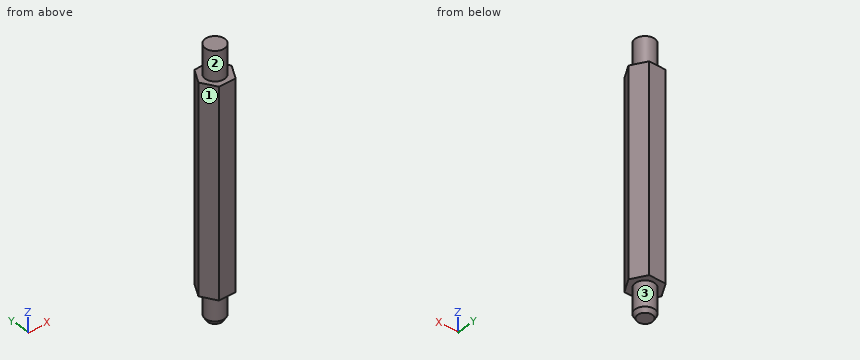
from build123d import *

# Parameters (mm, degrees)
EXTRUDE_1_DEPTH      = 42
EXTRUDE_2_DEPTH      = 6
EXTRUDE_2_DEPTH_BACK = 48
SKETCH_2_R           = 2
CHAMFER_1_SIZE       = 0.5
CHAMFER_1_SIZE2      = 0.866025404


with BuildPart() as part:
    # 草图1 → 拉伸1 (new body)
    with BuildSketch(Plane.XY):
        Polygon((1.732050808, -3), (3.464101615, 0), (1.732050808, 3), (-1.732050808, 3), (-3.464101615, 0), (-1.732050808, -3), align=None)
    extrude(amount=EXTRUDE_1_DEPTH)

    # 草图2 → 拉伸2 (add, two sides: drawn at the far end of the back side and taken through both)
    with BuildSketch(Plane.XY.offset(42).offset(-EXTRUDE_2_DEPTH_BACK)):
        with Locations(Location((0, 0, 0), (0, 0, 180))):
            Circle(SKETCH_2_R)
    extrude(amount=EXTRUDE_2_DEPTH + EXTRUDE_2_DEPTH_BACK)

    # 倒角1
    chamfer_1_edges = [part.edges().sort_by_distance(p)[0] for p in [
        (2, 0, -6),
    ]]
    chamfer_1_side = [part.faces().sort_by_distance(p)[0] for p in [
        (0, 0, -6),
    ]]
    chamfer(chamfer_1_edges, length=CHAMFER_1_SIZE, length2=CHAMFER_1_SIZE2, reference=chamfer_1_side[0])


solid = part.part
Design review of the part built by this model. Coordinates are the model's own, in mm. Face numbers are marked on the shaded views. A direction names the side the tool comes from. Round coordinates to 2 decimals unless told otherwise and drop trailing zeros. Loops run counter-clockwise (first coordinate to the right, second up) from the corner with the lowest first, then second, coordinate; pieces in that order, holes last. Notation, with made-up numbers: M 9,3.5 L 36,3.5 A24 cw 36,41.5 Z; hole C -39,70 d10. An arc over 180 degrees is marked long. Answer as a JSON object with one key per item and string values.
Item 1: We need section C-C on y = 2.5. Give the boundary of the cut face in (x, z).
Answer sheet:
{"outline": "M -2.02,0 L 2.02,0 L 2.02,42 L -2.02,42 Z"}
Item 2: We need section D-D on z = 45. Give the boundary of the cut face in (x, y).
Answer sheet:
{"outline": "C 0,0 d4"}
Item 3: Wall thickness on L1, parallel to Z at x = -2, y = 0.5; L2, parallel to X at y = 2.75, z = 21; L3, parallel to Y at x = 1.75, z = 27: over which ranges is each line inside the solid? List them lowest first. Write a range as from..to.
Answer sheet:
{"L1": "z = 0..42", "L2": "x = -1.88..1.88", "L3": "y = -2.97..2.97"}
Item 4: We need section B-B on z = 1.5. Give the boundary of the cut face in (x, y), and give its area (3 significant figures).
Answer sheet:
{"outline": "M -3.46,0 L -1.73,-3 L 1.73,-3 L 3.46,0 L 1.73,3 L -1.73,3 Z", "area": "31.2 mm^2"}
Item 5: Machinability: for the marked faces 1, 2 and 3, which of the approach directions +Z, -Z, +X, -X, +Y, -Y give a long, thin tool a straight path to every point of the face, cutting with its end or side? Answer none if there is none.
Answer sheet:
{"face 1": "+Z, -Z, -X, -Y", "face 2": "+Z", "face 3": "-Z"}
Item 6: We need section A-A on x = 0. Give the boundary of the cut face in (y, z), and give its area (3 significant figures).
Answer sheet:
{"outline": "M -3,0 L -2,0 L -2,-5.13 L -1.5,-6 L 1.5,-6 L 2,-5.13 L 2,0 L 3,0 L 3,42 L 2,42 L 2,48 L -2,48 L -2,42 L -3,42 Z", "area": "300 mm^2"}
